```python
from build123d import *

# Parameters (mm, degrees)
BOSS_EXTRU_1_DEPTH      = 4
ESQUISSE2_R             = 5.05
ESQUISSE2_R_2           = 3.5
ENL_V_MAT_EXTRU_1_DEPTH = 10
ENL_V_MAT_EXTRU_2_DEPTH = 2.5
ESQUISSE5_R             = 1.05
ENL_V_MAT_EXTRU_3_DEPTH = 51.225118218
CONG_2_R                = 1.5
CONG_3_R                = 10


with BuildPart() as part:
    # Esquisse1 → Boss.-Extru.1 (new body)
    with BuildSketch(Plane(origin=(0, 0, 0), x_dir=(0, 0, -1), z_dir=(1, 0, 0))):
        with BuildLine():
            Line((-33.755002002, 5), (20, 5))
            Line((20, 5), (38.152060387, 8.808241549))
            ThreePointArc((38.152060387, 8.808241549), (45.281301679, 7.28751347), (48.945833333, 0.985934061))
            ThreePointArc((48.945833333, 0.985934061), (49.25, 0), (48.945833333, -0.985934061))
            ThreePointArc((48.945833333, -0.985934061), (45.281301679, -7.28751347), (38.152060387, -8.808241549))
            Line((38.152060387, -8.808241549), (20, -5))
            Line((20, -5), (-33.755002002, -5))
            ThreePointArc((-33.755002002, -5), (-48, 0), (-33.755002002, 5))
        make_face()
    extrude(amount=BOSS_EXTRU_1_DEPTH)

    # Esquisse2 → Enlèv. mat.-Extru.1 (cut)
    with BuildSketch(Plane(origin=(4, 0, 0), x_dir=(0, 0, -1), z_dir=(1, 0, 0))):
        with Locations((-40, 0)):
            Circle(ESQUISSE2_R)
        with Locations((40, 0)):
            Circle(ESQUISSE2_R_2)
    extrude(amount=-ENL_V_MAT_EXTRU_1_DEPTH, mode=Mode.SUBTRACT)

    # Esquisse3 → Enlèv. mat.-Extru.2 (cut)
    with BuildSketch(Plane(origin=(4, 0, 0), x_dir=(0, 0, -1), z_dir=(1, 0, 0))):
        with BuildLine():
            Line((22.139192589, 2.473826593), (36.031373033, 4.5))
            ThreePointArc((36.031373033, 4.5), (46, 0), (36.031373033, -4.5))
            Line((36.031373033, -4.5), (22.139192589, -2.473826593))
            ThreePointArc((22.139192589, -2.473826593), (20, 0), (22.139192589, 2.473826593))
        make_face()
    extrude(amount=-ENL_V_MAT_EXTRU_2_DEPTH, mode=Mode.SUBTRACT)

    # Esquisse5 → Enlèv. mat.-Extru.3 (cut, through all)
    with BuildSketch(Plane(origin=(4, 0, 0), x_dir=(0, 0, -1), z_dir=(1, 0, 0))):
        with Locations((33.98959236, 6.01040764)):
            Circle(ESQUISSE5_R)
        with Locations(Location((33.98959236, -6.01040764, 0), (0, 0, 180))):
            Circle(ESQUISSE5_R)
        with Locations((47.5, 0)):
            Circle(ESQUISSE5_R)
    extrude(amount=-ENL_V_MAT_EXTRU_3_DEPTH, mode=Mode.SUBTRACT)

    # Congé2
    cong_2_edges = [part.edges().sort_by_distance(p)[0] for p in [
        (2, -0.985934061, -48.945833333),
        (2, -5, -20),
        (2, 5, -20),
        (2, 0.985934061, -48.945833333),
    ]]
    fillet(cong_2_edges, radius=CONG_2_R)

    # Congé3
    cong_3_edges = [part.edges().sort_by_distance(p)[0] for p in [
        (2, -5, 33.755002002),
        (2, 5, 33.755002002),
    ]]
    fillet(cong_3_edges, radius=CONG_3_R)


solid = part.part
```
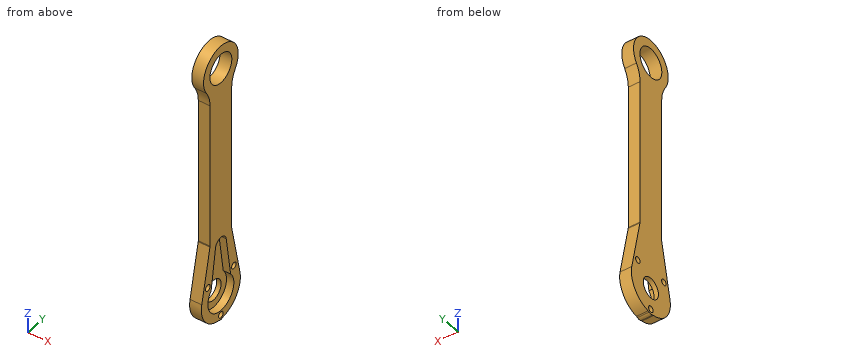
The listing builds one solid part. Answer for the finished solid, in the listing's coordinates (mm). Coordinates: 2 decimals unless noted, no trailing zeros. Write each loop counter-clockwise with the first axis right and the second up, starting at its lowest first coordinate (ties: lowest second). Pieces come first, ordered by that corner, then holes. Notation, with made-up numbers: (-19.5, 45.5) - (-10.5, 45.5) arc R18 ccw to (-10.5, 58.5) - close; hole circle Ø2 at (-19, 85.5). An arc over 180 degrees is marked (long way). Return JSON: item names as keys, results as strings. Group by question number.
Q1. The part is cut by section B-B on z = 40. Write down the section's boundary in (x, y).
Q2. The part is cut by section D-D on z = 0.5. Write down the section's boundary in (x, y), and give its area (3 significant figures).
Q3. The part is cut by section A-A on y = 0. Write down the section's boundary in (x, z).
Q4. Find the intervals of material crossed by line 1 along Y through (x, z) = (3.4, -40); line 2 along Z through (x, y) = (3.5, 0.75); line 3 along Z through (x, y) = (1.15, 0.5), in increasing order. Write a range as [from, to].
Q5. The part is cut by section C-C on z = -40. Write down the section's boundary in (x, y), and give its area (3 significant figures).
Q6. Flat-ended cylindrical pins translate along their axes: pin 1 Ø1.2 at (x, z) = (2, 0.5) entering from -Y; pin 2 Ø8 at (y, z) = (0, -40) entering from +X. Find the tip coordinate at first contact, or state that the pin passes through.
Evaluation:
{
 "1": {"outline": "(0, -8) - (4, -8) - (4, -5.05) - (0, -5.05) - close; (0, 5.05) - (4, 5.05) - (4, 8) - (0, 8) - close"},
 "2": {"outline": "(0, -5) - (4, -5) - (4, 5) - (0, 5) - close", "area": "40.0 mm2"},
 "3": {"outline": "(0, -49.25) - (4, -49.25) - (4, -48.55) - (0, -48.55) - close; (0, -46.45) - (4, -46.45) - (4, -46) - (1.5, -46) - (1.5, -43.5) - (0, -43.5) - close; (0, -36.5) - (1.5, -36.5) - (1.5, -20) - (4, -20) - (4, 34.95) - (0, 34.95) - close; (0, 45.05) - (4, 45.05) - (4, 48) - (0, 48) - close"},
 "4": {"line 1": "y = [-9, -6], [6, 9]", "line 2": "z = [-49.08, -48.23], [-46.77, -45.95], [-20.12, 35.01], [44.99, 47.96]", "line 3": "z = [-49.18, -48.42], [-46.58, -43.46], [-36.54, 34.97], [45.03, 47.98]"},
 "5": {"outline": "(0, -9) - (4, -9) - (4, -6) - (1.5, -6) - (1.5, -3.5) - (0, -3.5) - close; (0, 3.5) - (1.5, 3.5) - (1.5, 6) - (4, 6) - (4, 9) - (0, 9) - close", "area": "31.5 mm2"},
 "6": {"pin 1": "stops at y = -5", "pin 2": "stops at x = 1.5"}
}
